Read the model definition and answer for the solid it produces. Units are mm, in the model's axes. A direction names the side the tool comes from. Round coordinates to 2 decimals unless told otherwise and drop trailing zeros. Loops run counter-clockwise (first coordinate to the right, second up) from the corner with the lowest first, then second, coordinate; pieces in that order, holes last. Notation, with made-up numbers: M -22.5,-23 L 21.5,-23 A8 ccw 21.5,-13 Z; hole C 78.25,-13.75 d8. An arc over 180 degrees is marked long. Answer as CSV lines item,"result".
```python
from build123d import *

# Parameters (mm, degrees)
CROQUIS1_R              = 3
CROQUIS1_R_2            = 5
SALIENTE_EXTRUIR1_DEPTH = 3


with BuildPart() as part:
    # Croquis1 → Saliente-Extruir1 (new body)
    with BuildSketch(Plane(origin=(0, 0, 0), x_dir=(1, 0, 0), z_dir=(0, 1, 0))):
        Polygon((0, 3), (110, 3), (110, 12.5), (107, 12.5), (107, 20), (107, 27.5), (110, 27.5), (110, 37), (110, 140), (89.5, 140), (20.5, 140), (0, 140), (0, 50), (0, 35), (3, 35), (3, 20), (3, 15), (0, 15), align=None)
        with Locations(Location((10.25, 60.5, 0), (0, 0, 270))):
            Circle(CROQUIS1_R, mode=Mode.SUBTRACT)
        with Locations(Location((85, 20, 0), (0, 0, 270))):
            Circle(CROQUIS1_R_2, mode=Mode.SUBTRACT)
        with Locations(Location((99.75, 60.5, 0), (0, 0, 270))):
            Circle(CROQUIS1_R, mode=Mode.SUBTRACT)
        with Locations(Location((10.25, 99.5, 0), (0, 0, 270))):
            Circle(CROQUIS1_R, mode=Mode.SUBTRACT)
        Polygon((92.5, 37), (89.5, 37), (20.5, 37), (17.5, 37), (17.5, 40), (20.5, 40), (20.5, 71), (17.5, 71), (17.5, 72.5), (14.5, 72.5), (14.5, 75.5), (17.5, 75.5), (17.5, 77), (20.5, 77), (20.5, 83), (17.5, 83), (17.5, 84.5), (14.5, 84.5), (14.5, 87.5), (17.5, 87.5), (17.5, 89), (20.5, 89), (20.5, 130), (89.5, 130), (89.5, 89), (89.5, 71), (89.5, 40), (92.5, 40), align=None, mode=Mode.SUBTRACT)
        with Locations(Location((99.75, 99.5, 0), (0, 0, 270))):
            Circle(CROQUIS1_R, mode=Mode.SUBTRACT)
    extrude(amount=SALIENTE_EXTRUIR1_DEPTH)


solid = part.part
```
1) Each of these flat-tipped pins is pushed along its axis until it touches: P1, Ø5, axis at x = 99.75, z = -60.5, coming from the -Y side; P2, Ø1, axis at y = 2.5, z = -63, coming from the -X side. Where does it stop, or does it pass through?
Evaluation:
P1,"passes through"
P2,"stops at x = 0"
2) Determine the mould class of faces 1 (the flat face through (20.5, 1, -80)), 2 (the flat face through (91, 3, -72)), 3 (the flat face through (56, 1, -140)), 4 (the cylindrical face through (10.382, 1.479, -102.497)) for opening direction Z: released by +Z, released by -Z, zero draft, split by the parting line, or undercut.
Evaluation:
face 1,"undercut"
face 2,"zero draft"
face 3,"released by -Z"
face 4,"undercut"
3) A tool of negligible diameter and unlimited length cuts with its end or side. For faces 5 (the flat face through (2, 1, -15)), 6 (the flat face through (20.5, 1, -55)), 7 (the flat face through (108, 1, -27.5)), from which of +Z, -Z, +X, -X, +Y, -Y can it reach the whole face along a straight path? Write none if from no direction.
Evaluation:
face 5,"-X, +Y, -Y"
face 6,"+Y, -Y"
face 7,"+X, +Y, -Y"
4) Find section A-A, the plane x = 85. Give the vertices of the cut face in (y, z).
Evaluation:
outline,"M 0,-140 L 3,-140 L 3,-130 L 0,-130 Z; M 0,-37 L 3,-37 L 3,-25 L 0,-25 Z; M 0,-15 L 3,-15 L 3,-3 L 0,-3 Z"
5) Find section B-B, the plane z = -60.5. Give the vertices of the cut face in (x, y), then the cut area to 3 significant figures.
Evaluation:
outline,"M 0,0 L 7.25,0 L 7.25,3 L 0,3 Z; M 13.25,0 L 20.5,0 L 20.5,3 L 13.25,3 Z; M 89.5,0 L 96.75,0 L 96.75,3 L 89.5,3 Z; M 102.75,0 L 110,0 L 110,3 L 102.75,3 Z"
area,"87.0 mm^2"
6) Find section C-C, the plane x = 72. Give the vertices of the cut face in (y, z), then the cut area to 3 significant figures.
Evaluation:
outline,"M 0,-140 L 3,-140 L 3,-130 L 0,-130 Z; M 0,-37 L 3,-37 L 3,-3 L 0,-3 Z"
area,"132 mm^2"
7) Find section D-D, the plane z = -86. Give the vertices of the cut face in (x, y), then the cut area to 3 significant figures.
Evaluation:
outline,"M 0,0 L 14.5,0 L 14.5,3 L 0,3 Z; M 89.5,0 L 110,0 L 110,3 L 89.5,3 Z"
area,"105 mm^2"
8) Straight lines are drawn through the part: line 1 (X direction, y = 1, z = -60.5); line 2 (X direction, y = 0.8, z = -20); line 3 (Z direction, x = 10.5, y = 0.55). For each, find the intervals that lie inside material, in ascending order.
Evaluation:
line 1,"x = 0 to 7.25, 13.25 to 20.5, 89.5 to 96.75, 102.75 to 110"
line 2,"x = 3 to 80, 90 to 107"
line 3,"z = -140 to -102.49, -96.51 to -63.49, -57.51 to -3"
